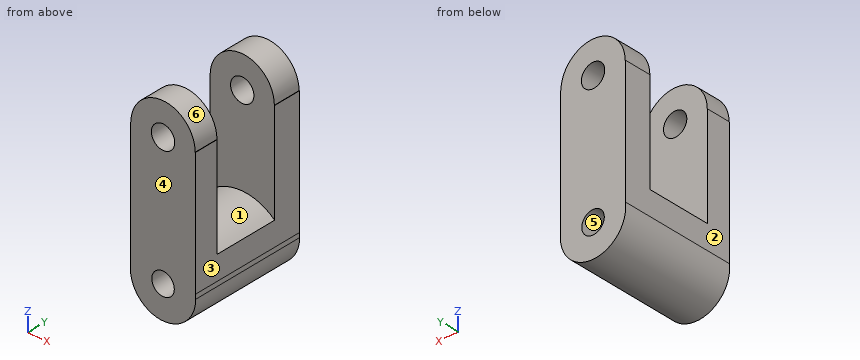
from build123d import *

# Parameters (mm, degrees)
F1_DEPTH = 76.2
F2_W     = 42.1064179391
F2_H     = 26.5092402697
F2_H_2   = 66.0529509187
F3_DEPTH = 127
F5_DEPTH = 45.72


with BuildPart() as f1:
    # F0 (on Front) → F1 (new body)
    with BuildSketch(Plane.XZ):
        with BuildLine():
            ThreePointArc((-10.6776429778, 46.1808890104), (-3.0418550596, 53.8166769287), (4.5939328587, 46.1808890104))
            Line((4.5939328587, 46.1808890104), (17.9729815764, 46.1808890104))
            ThreePointArc((17.9729815764, 46.1808890104), (-3.0418550596, 67.1957256464), (-24.0566916955, 46.1808890104))
            Line((-24.0566916955, 46.1808890104), (-10.6776429778, 46.1808890104))
        make_face()
        with BuildLine():
            Line((17.9729815764, 46.1808890104), (4.5939328587, 46.1808890104))
            ThreePointArc((4.5939328587, 46.1808890104), (-3.0418550596, 38.5451010922), (-10.6776429778, 46.1808890104))
            Line((-10.6776429778, 46.1808890104), (-24.0566916955, 46.1808890104))
            ThreePointArc((-24.0566916955, 46.1808890104), (-3.0418550596, 25.1660523745), (17.9729815764, 46.1808890104))
        make_face()
        with BuildLine():
            Line((18.1589517742, 46.1808890104), (17.9729815764, 46.1808890104))
            ThreePointArc((17.9729815764, 46.1808890104), (-3.0418550596, 25.1660523745), (-24.0566916955, 46.1808890104))
            Line((-24.0566916955, 46.1808890104), (-24.2426618934, 46.1808890104))
            Line((-24.2426618934, 46.1808890104), (-24.2426618934, -35.4456115543))
            ThreePointArc((-24.2426618934, -35.4456115543), (-3.0418550596, -16.8676737579), (18.1589517742, -35.4456115543))
            Line((18.1589517742, -35.4456115543), (18.1589517742, 46.1808890104))
        make_face()
        with BuildLine():
            Line((18.1589517742, -38.2536314428), (18.1589517742, -35.4456115543))
            ThreePointArc((18.1589517742, -35.4456115543), (-3.0418550596, -16.8676737579), (-24.2426618934, -35.4456115543))
            Line((-24.2426618934, -35.4456115543), (-24.2426618934, -38.2536314428))
            Line((-24.2426618934, -38.2536314428), (-10.4049137752, -38.2536314428))
            ThreePointArc((-10.4049137752, -38.2536314428), (-3.0418550596, -30.8905727272), (4.321203656, -38.2536314428))
            Line((4.321203656, -38.2536314428), (18.1589517742, -38.2536314428))
        make_face()
        with BuildLine():
            ThreePointArc((18.3441026253, -38.2536314428), (18.2977647113, -36.8465727614), (18.1589517742, -35.4456115543))
            Line((18.1589517742, -35.4456115543), (18.1589517742, -38.2536314428))
            Line((18.1589517742, -38.2536314428), (4.321203656, -38.2536314428))
            ThreePointArc((4.321203656, -38.2536314428), (-3.0418550596, -45.6166901584), (-10.4049137752, -38.2536314428))
            Line((-10.4049137752, -38.2536314428), (-24.2426618934, -38.2536314428))
            Line((-24.2426618934, -38.2536314428), (-24.2426618934, -35.4456115543))
            ThreePointArc((-24.2426618934, -35.4456115543), (-4.448913741, -59.5932512137), (18.3441026253, -38.2536314428))
        make_face()
    extrude(amount=F1_DEPTH)

    # F2 (on face) → F3 (cut)
    with BuildSketch(Plane.YZ.offset(18.1589517742)):
        with Locations((-39.1769716516, 59.4355091453)):
            Rectangle(F2_W, F2_H)
        with Locations((-39.1769716516, 13.1544135511)):
            Rectangle(F2_W, F2_H_2)
    extrude(amount=-F3_DEPTH, mode=Mode.SUBTRACT)

    # F4 (on face) → F5 (join)
    with BuildSketch(Plane.XZ.offset(18.1237626821)):
        with BuildLine():
            Line((-24.2426618934, -19.8720619082), (18.1589517742, -19.8720619082))
            ThreePointArc((18.1589517742, -19.8720619082), (-3.0418550596, -11.8207453955), (-24.2426618934, -19.8720619082))
        make_face()
    extrude(amount=F5_DEPTH)


solid = f1.part
Part model, mm, in its own coordinate system. Face numbers are marked on the shaded views. A direction names the side the tool comes from. Coordinates: 2 decimals unless noted, no trailing zeros. Write each loop counter-clockwise with the first axis right and the second up, starting at its lowest first coordinate (ties: lowest second). Pieces come first, ordered by that corner, then holes. Notation, with made-up numbers: M 31.25,82.25 L 90.25,82.25 A11 ccw 90.25,92.25 Z; hole C 31.5,-35 d3. An arc over 180 degrees is marked long. Return JSON: item names as keys, results as strings.
1. Pull direction X, two halves, no side cores. Call the marked faces 4, 5 and 6: pulls with the +X half, pulls with the -X half, needs draft (parallel to the pull), parting line crosses it, or undercut.
Determined:
{"face 4": "needs draft", "face 5": "undercut", "face 6": "parting line crosses it"}
2. Saw through at D-D, the plane y = -31. Write the cut outline in (x, z).
Determined:
{"outline": "M -24.24,-35.45 A21.39 ccw long 18.16,-35.45 L 18.16,-19.87 A31.94 ccw -24.24,-19.87 Z; hole C -3.04,-38.25 d14.73"}
3. Saw through at A-A, the plane y = -15. Write the cut outline in (x, z).
Determined:
{"outline": "M -24.24,-35.45 A21.39 ccw long 18.16,-35.45 L 18.16,46.18 L 17.97,46.18 A21.01 ccw -24.06,46.18 L -24.24,46.18 Z; hole C -3.04,46.18 d15.27; hole C -3.04,-38.25 d14.73"}
4. Saw through at B-B, the plane x = -1.5. Write the cut outline in (y, z), then the cut area to 3 significant figures.
Determined:
{"outline": "M -76.2,-59.58 L 0,-59.58 L 0,-45.45 L -76.2,-45.45 Z; M -76.2,-31.05 L 0,-31.05 L 0,38.7 L -18.12,38.7 L -18.12,-11.86 L -60.23,-11.86 L -60.23,38.7 L -76.2,38.7 Z; M -76.2,53.66 L -60.23,53.66 L -60.23,67.14 L -76.2,67.14 Z; M -18.12,53.66 L 0,53.66 L 0,67.14 L -18.12,67.14 Z", "area": "4,720 mm²"}
5. Probe L1, parallel to Y at x = 15, z = 36; L2, parallel to Z at x = -1.5, y = -8; L3, parallel to Z at x = -9, y = -7. List the from-to ranges inside material, lowest first.
Determined:
{"L1": "-76.2 to -60.23, -18.12 to 0", "L2": "-59.58 to -45.45, -31.05 to 38.7, 53.66 to 67.14", "L3": "-58.79 to -42.58, -33.93 to 41.41, 50.96 to 66.33"}
6. Flat gauge pins, fed straight in: pin 1 Ø4 at (y, z) = (-8, 38) entering from -X; pin 2 Ø2 at (x, y) = (8, -26.5) entering from -Z; pin 3 Ø1.5 at (y, z) = (-67, 30) entering from +X; pin 4 Ø9 at (x, z) = (-3.04, 46.18) entering from +Y. Where does each tip first touch, or does it go through?
Determined:
{"pin 1": "x = -24.24", "pin 2": "z = -57.14", "pin 3": "x = 18.16", "pin 4": "through"}
7. 3-axis set-ups, long thin cutter, end or side, ignore diameter. For the marked faces 1, 2 and 3: which of +Z, -Z, +X, -X, +Y, -Y reach the whole face in a straight line?
Determined:
{"face 1": "+Z", "face 2": "+Z, -X, +Y, -Y", "face 3": "+Z, +X, +Y, -Y"}
8. Saw through at C-C, the plane z = -6. Write the cut outline in (x, y), then the cut area to 3 significant figures.
Determined:
{"outline": "M -24.24,-76.2 L 18.16,-76.2 L 18.16,-60.23 L -24.24,-60.23 Z; M -24.24,-18.12 L 18.16,-18.12 L 18.16,0 L -24.24,0 Z", "area": "1,450 mm²"}
